Geometry: final body of the model. Coordinates: model frame, mm. Face numbers are marked on the shaded views. A direction names the side the tool comes from. Give positions to 0.01 mm unless a question says otherwise; leave off trailing zeros. Loops run counter-clockwise (first coordinate to the right, second up) from the corner with the lowest first, then second, coordinate; pieces in that order, holes last. Notation, with made-up numbers: (47.5, 58.5) - (106.5, 58.5) arc R22 ccw to (106.5, 78.5) - close; hole circle Ø6 at (67, -2). An arc over 180 degrees is marked (long way). Answer in a Markdown table with one row per item.
from build123d import *

# Parameters (mm, degrees)
SKETCH_1_W          = 40
SKETCH_1_H          = 39
EXTRUDE_1_DEPTH     = 20
SKETCH_2_W          = 20
SKETCH_2_H          = 5
EXTRUDE_2_DEPTH     = 8
SKETCH_3_R          = 2
CUT_EXTRUDE_1_DEPTH = 8
SKETCH_4_R          = 7.5
EXTRUDE_3_DEPTH     = 1.5
SKETCH_5_R          = 6
EXTRUDE_4_DEPTH     = 0.5
SKETCH_6_R          = 3
EXTRUDE_5_DEPTH     = 4
FILLET_1_R          = 1


with BuildPart() as part:
    # 草图1 → 凸台-拉伸1 (new body)
    with BuildSketch(Plane.XY):
        Rectangle(SKETCH_1_W, SKETCH_1_H)
    extrude(amount=EXTRUDE_1_DEPTH)

    # 草图2 → 凸台-拉伸2 (add)
    with BuildSketch(Plane(origin=(20, 0, 0), x_dir=(0, 0, -1), z_dir=(1, 0, 0))):
        with Locations((-10, 9)):
            Rectangle(SKETCH_2_W, SKETCH_2_H)
    extrude_2 = extrude(amount=EXTRUDE_2_DEPTH)

    # 草图3 → 切除-拉伸1 (cut)
    with BuildSketch(Plane(origin=(0, 11.5, 0), x_dir=(1, 0, 0), z_dir=(0, 1, 0))):
        with Locations(Location((24, -4.678896128, 0), (0, 0, 180))):
            Circle(SKETCH_3_R)
        with Locations(Location((24, -14.678896128, 0), (0, 0, 180))):
            Circle(SKETCH_3_R)
    cut_extrude_1 = extrude(amount=-CUT_EXTRUDE_1_DEPTH, mode=Mode.SUBTRACT)

    # 镜向1: 凸台-拉伸2, 切除-拉伸1 across plane
    add(extrude_2.mirror(Plane(origin=(0, 0, 0), x_dir=(0, 0, 1), z_dir=(1, 0, 0))))
    add(cut_extrude_1.mirror(Plane(origin=(0, 0, 0), x_dir=(0, 0, 1), z_dir=(1, 0, 0))), mode=Mode.SUBTRACT)

    # 草图4 → 凸台-拉伸3 (add)
    with BuildSketch(Plane(origin=(0, 19.5, 0), x_dir=(1, 0, 0), z_dir=(0, 1, 0))):
        with Locations(Location((-10, -9.678896128, 0), (0, 0, 90))):
            Circle(SKETCH_4_R)
    extrude(amount=EXTRUDE_3_DEPTH)

    # 草图5 → 凸台-拉伸4 (add)
    with BuildSketch(Plane(origin=(0, 21, 0), x_dir=(1, 0, 0), z_dir=(0, 1, 0))):
        with Locations(Location((-10, -9.678896128, 0), (0, 0, 270))):
            Circle(SKETCH_5_R)
    extrude(amount=EXTRUDE_4_DEPTH)

    # 草图6 → 凸台-拉伸5 (add)
    with BuildSketch(Plane(origin=(0, 21.5, 0), x_dir=(1, 0, 0), z_dir=(0, 1, 0))):
        with Locations(Location((-10, -9.678896128, 0), (0, 0, 270))):
            Circle(SKETCH_6_R)
    extrude(amount=EXTRUDE_5_DEPTH)

    # 圆角1
    fillet_1_edges = [part.edges().sort_by_distance(p)[0] for p in [
        (-20, 15.5, 20),
        (20, 15.5, 0),
        (20, 15.5, 20),
        (0, -19.5, 20),
        (28, 9, 20),
        (28, 9, 0),
        (-20, -6.5, 0),
        (-20, -6.5, 20),
        (-28, 9, 20),
        (-28, 9, 0),
        (20, -6.5, 20),
        (0, -19.5, 0),
        (-20, 15.5, 0),
        (0, 19.5, 0),
        (20, -6.5, 0),
        (20, -19.5, 10),
        (-20, -19.5, 10),
        (-20, 19.5, 10),
        (20, 19.5, 10),
        (0, 19.5, 20),
    ]]
    fillet(fillet_1_edges, radius=FILLET_1_R)


solid = part.part
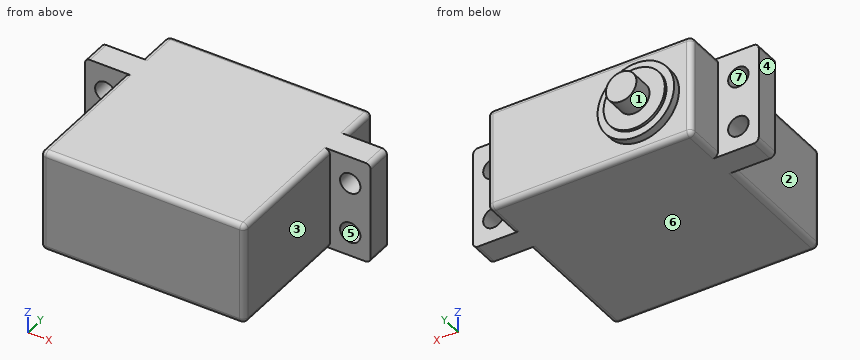
Q1. Cut plane A-A (x = 24). Output: boundary loops of the cut face in (y, z), and give its area (3 significant figures).
Check values:
| item | result |
|---|---|
| outline | (6.5, 0) - (11.5, 0) - (11.5, 2.68) - (6.5, 2.68) - close; (6.5, 6.68) - (11.5, 6.68) - (11.5, 12.68) - (6.5, 12.68) - close; (6.5, 16.68) - (11.5, 16.68) - (11.5, 20) - (6.5, 20) - close |
| area | 60.0 mm² |
Q2. Draft query along Z for the marked faces 4, 5, 6 and 7. Return one class per face: pulls with the +Z half, pulls with the -Z half, needs draft (parallel to the pull), parting line crosses it, or undercut.
Check values:
| item | result |
|---|---|
| face 4 | needs draft |
| face 5 | undercut |
| face 6 | pulls with the -Z half |
| face 7 | undercut |
Q3. Reachability of the marked faces 1, 2 and 3 from +Z, -Z, +X, -X, +Y, -Y: full face, straight path, thin tool, end or side. Return the list, or none.
Check values:
| item | result |
|---|---|
| face 1 | +Y |
| face 2 | +Z, -Z, -X, -Y |
| face 3 | +Z, -Z, +X, -Y |
Q4. Material intervals for line 1 along Z through (x, y) = (-24, 8.85); line 2 along Y through (x, z) = (-7, 6.5); line 3 along Y through (x, z) = (16, 6.25), sorted ascending.
Check values:
| item | result |
|---|---|
| line 1 | 0 to 2.68, 6.68 to 12.68, 16.68 to 20 |
| line 2 | -19.5 to 21.5 |
| line 3 | -19.5 to 19.5 |
Q5. Cut plane D-D (z = 9). Output: boundary loops of the cut face in (x, y).
Check values:
| item | result |
|---|---|
| outline | (-28, 6.5) - (-20, 6.5) - (-20, -18.5) arc R1 ccw to (-19, -19.5) - (19, -19.5) arc R1 ccw to (20, -18.5) - (20, 6.5) - (28, 6.5) - (28, 11.5) - (20, 11.5) - (20, 18.5) arc R1 ccw to (19, 19.5) - (-2.53, 19.5) - (-2.53, 21) - (-4.04, 21) - (-4.04, 21.5) - (-7.08, 21.5) - (-7.08, 25.5) - (-12.92, 25.5) - (-12.92, 21.5) - (-15.96, 21.5) - (-15.96, 21) - (-17.47, 21) - (-17.47, 19.5) - (-19, 19.5) arc R1 ccw to (-20, 18.5) - (-20, 11.5) - (-28, 11.5) - close |
Q6. Cut plane B-B (x = -1.5). Output: boundary loops of the cut face in (y, z), and give its area (3 significant figures).
Check values:
| item | result |
|---|---|
| outline | (-19.5, 1) arc R1 ccw to (-18.5, 0) - (18.5, 0) arc R1 ccw to (19.5, 1) - (19.5, 19) arc R1 ccw to (18.5, 20) - (-18.5, 20) arc R1 ccw to (-19.5, 19) - close |
| area | 779 mm² |
Q7. Cut plane C-C (y = -2). Output: boundary loops of the cut face in (x, z).
Check values:
| item | result |
|---|---|
| outline | (-20, 1) arc R1 ccw to (-19, 0) - (19, 0) arc R1 ccw to (20, 1) - (20, 19) arc R1 ccw to (19, 20) - (-19, 20) arc R1 ccw to (-20, 19) - close |
Q8. First-contact query: pin 1 (10 mm diameter, centred on x = 21.5, z = 9, fed in from +Y); pin 2 (2.5 mm diameter, centred on x = -23, z = 12.5, fed in from +Y); pin 3 (2 mm diameter, centred on y = 13.5, z = 10, fed in from -X). Flat tips, straight axial feed; report the tip coordinate or a pass-through.
Check values:
| item | result |
|---|---|
| pin 1 | y = 19.5 |
| pin 2 | y = 11.5 |
| pin 3 | x = -20 |
